For this review, take the finished solid that the model builds, in its own axes (mm). A direction names the side the tool comes from. Coordinates: 2 decimals unless noted, no trailing zeros. Order: outer loops, then holes, each group sorted by start corner. A loop starts at its lowest first (then second) coordinate and runs counter-clockwise, first axis right, second up. Notation, with made-up numbers: (24.5, 74.25) -> (77.5, 74.25) arc R28 cw to (77.5, 107.25) -> close; hole circle Ø8 at (36, 85.25). An arc over 180 degrees is marked (long way). Write item = value, one per line. Start each with the question number.
1) Insertion check: pin 1 Ø10 at (x, y) = (136, -16.5) entering from -Z (3 decimals); pin 2 Ø6 at (x, y) = (159, 22) entering from +Z; pin 3 Ø20 at (x, y) = (-22.5, 6) entering from -Z. Each pin has a flat end and moves straight along its axis. Give the tip position at first contact, or say it passes through.
2) Wall thickness on probe 1 along X at (y, z) = (9, -31.5); probe 2 along Y at (x, z) = (93.5, -4); probe 3 along Z at (x, y) = (72, 24.5): over which ranges is each line inside the solid? List them lowest first. Write a range as [from, to].
3) Consider section D-D on x = 153. Give the boundary of the cut face in (y, z), and give its area (3 significant figures).
4) Consider section A-A on x = -14. Give the boundary of the cut face in (y, z), and give its area (3 significant figures).
5) Machinability: for faces 1 (the face through (-20, -22, -23)), 2 (the face through (-20, 0, -25)), 3 (the face through (-20, 22, -23)), 4 (the face through (69.72, -1.32, 29.97)), 5 (the face through (-20, 0, 25)), which of the approach directions +Z, -Z, +X, -X, +Y, -Y give a long, thin tool a straight path to every point of the face, cutting with its end or side? Answer none if there is none.
6) Consider section B-B on y = 0. Give the boundary of the cut face in (x, z), and give its area (3 significant figures).
Autodesk Fusion 360 part; units mm, degrees
sketch "Sketch1" plane through (0, 0, 0) normal (0, 1, 0) x (1, 0, 0) in component "Shaft02"
  line L0 (0, 0) -> (0, 40)
  line L1 (0, 40) -> (10, 50)
  line L2 (0, 40) -> (22.4585, 40) construction
  line L3 (10, 50) -> (10, 0)
  line L4 (0, 0) -> (50, 0)
  line L5 (50, 0) -> (50, 30)
  line L6 (10, 50) -> (20, 50)
  line L7 (20, 50) -> (50, 30)
  line L8 (50, 0) -> (90, 0)
  line L9 (90, 0) -> (90, 30)
  line L10 (90, 30) -> (50, 30)
  line L11 (50, 30) -> (50, 0)
  line L12 (90, 0) -> (100, 0)
  line L13 (90, 30) -> (100, 22)
  line L14 (100, 0) -> (216, 0)
  line L15 (216, 0) -> (216, 22)
  line L16 (216, 22) -> (100, 22)
  line L17 (100, 22) -> (100, 0)
  dimension "d2" = 40
  dimension "d3" = 45
  dimension "d5" = 50
  dimension "d6" = 50
  dimension "d7" = 30
  dimension "d8" = 10
  dimension "d10" = 40
  dimension "d11" = 30
  dimension "d13" = 10
  dimension "d15" = 116
  dimension "d16" = 22
revolve "Revolve1" add sketch "Sketch1" angle 360 about axis through (100, 0, 0) along (1, 0, 0) in component "Shaft02"
sketch "Sketch2" plane through (0, 0, 0) normal (-1, 0, 0) x (0, -1, 0) in component "Shaft02"
  circle A0 centre (0, 0) radius 40
  line L0 (25, -25) -> (-25, -25)
  line L1 (-25, -25) -> (-25, 25)
  line L2 (-25, 25) -> (25, 25)
  line L3 (25, 25) -> (25, -25)
  line L4 (25, -25) -> (-25, 25) construction
  line L5 (-25, -25) -> (25, 25) construction
  dimension "d19" = 50
  dimension "d20" = 50
extrude "Extrude1" add sketch "Sketch2" along normal blind 40 contours L0 L1 L2 L3 in component "Shaft02"
chamfer "Chamfer1" distance 5 angle 45 4 edges at (-20, -25, 25) (-20, 25, 25) (-20, -25, -25) (-20, 25, -25) in component "Shaft02"
fillet "Fillet1" radius 5 1 edges at (216, -7.9555, 20.5112) in component "Shaft02"
component "Shaft02" placed x (1, 0, 0) y (0, 1, 0) z (0, 0, 1) at (0, 0, 0)
Answer sheet:
q1.pin_1 = -18.755
q1.pin_2 = 11.09
q1.pin_3 = -25
q2.probe_1 = [0, 45.86]
q2.probe_2 = [-26.9, 26.9]
q2.probe_3 = [-17.31, 17.31]
q3.outline = circle Ø44 at (0, 0)
q3.area = 1,520 mm2
q4.outline = (-25, -20) -> (-20, -25) -> (20, -25) -> (25, -20) -> (25, 20) -> (20, 25) -> (-20, 25) -> (-25, 20) -> close
q4.area = 2,450 mm2
q5.face_1 = -Z, -X, -Y
q5.face_2 = -Z, -X, +Y, -Y
q5.face_3 = -Z, -X, +Y
q5.face_4 = +X
q5.face_5 = +Z, -X, +Y, -Y
q6.outline = (-40, -25) -> (0, -25) -> (0, -40) -> (10, -50) -> (20, -50) -> (50, -30) -> (90, -30) -> (100, -22) -> (211, -22) arc R5 ccw to (216, -17) -> (216, 17) arc R5 ccw to (211, 22) -> (100, 22) -> (90, 30) -> (50, 30) -> (20, 50) -> (10, 50) -> (0, 40) -> (0, 25) -> (-40, 25) -> close
q6.area = 14,300 mm2
